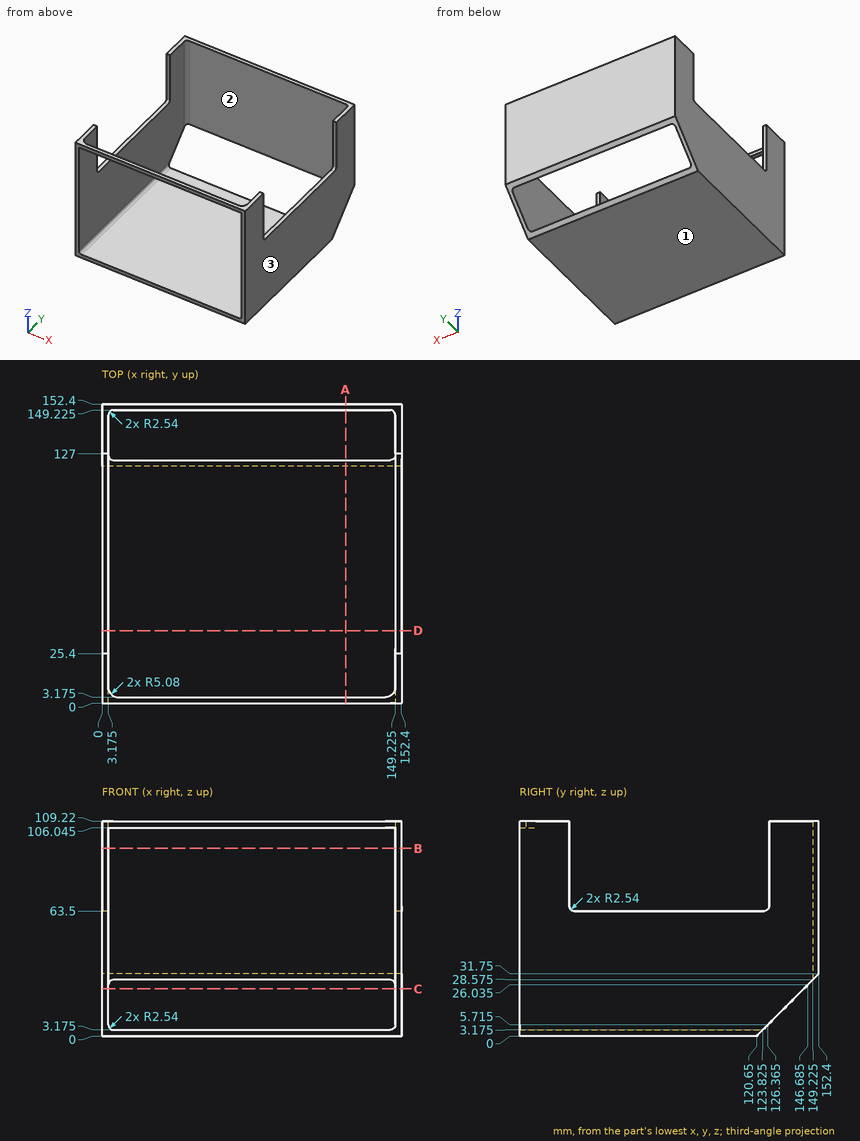
Answer from the drawing. Dimensions are ordinates in mm from the lowest x, y and z of the part. Coordinates: 2 decimals unless noted, no trailing zeros. Loops run counter-clockwise (first coordinate to the right, second up) from the corner with the lowest first, then second, coordinate; pieces in that order, holes last.
Q1. The part is cut by section A-A on x = 124. Write down the section's boundary in (y, z) (3 decimals).
Q2. The part is cut by section C-C on z = 24. Write down the section's boundary in (x, y) (3 decimals).
Q3. Each of these flat-tipped pins is pushed along its axis until it touches: pin 1 Ø2.5 at (x, y) = (1.5, 56) entering from +Z; pin 2 Ø12 at (x, z) = (124.5, 45.5) entering from -Y (3 decimals). Where does it stop, or does it pass through?
Q4. Consider probe 1 along X at (y, z) = (77, 32) (3 decimals); probe 2 along Z at (x, y) = (82.5, 10) (3 decimals); probe 3 along Y at (x, z) = (145, 65) (3 decimals). Determine where each line is inside the solid, lowest interval first.
Q5. The part is cut by section D-D on y = 37. Write down the section's boundary in (x, z) (3 decimals).
Q6. The mould has two halves that part along X. Classify the marked faces 1, 2 and 3: +X half, -X half, draft (parallel to the pull), parting line (faces both ways), or undercut.
Q7. The part is cut by section B-B on z = 95.5. Write down the section's boundary in (x, y) (3 decimals), and give its area (3 significant figures).
Results below:
1. outline: (0, 0) - (120.65, 0) - (123.825, 3.175) - (0, 3.175) - close; (0, 106.045) - (3.175, 106.045) - (3.175, 109.22) - (0, 109.22) - close; (149.225, 28.575) - (152.4, 31.75) - (152.4, 109.22) - (149.225, 109.22) - close
2. outline: (0, 0) - (3.175, 0) - (3.175, 144.65) - (0, 144.65) - close; (149.225, 0) - (152.4, 0) - (152.4, 144.65) - (149.225, 144.65) - close
3. pin 1: stops at z = 63.5
3. pin 2: stops at y = 149.225
4. probe 1: x = 0 to 3.175, 149.225 to 152.4
4. probe 2: z = 0 to 3.175
4. probe 3: y = 149.225 to 152.4
5. outline: (0, 0) - (152.4, 0) - (152.4, 63.5) - (149.225, 63.5) - (149.225, 5.715) arc R2.54 cw to (146.685, 3.175) - (5.715, 3.175) arc R2.54 cw to (3.175, 5.715) - (3.175, 63.5) - (0, 63.5) - close
6. face 1: draft
6. face 2: undercut
6. face 3: +X half
7. outline: (0, 0) - (3.175, 0) - (3.175, 25.4) - (0, 25.4) - close; (0, 127) - (3.175, 127) - (3.175, 146.685) arc R2.54 cw to (5.715, 149.225) - (146.685, 149.225) arc R2.54 cw to (149.225, 146.685) - (149.225, 127) - (152.4, 127) - (152.4, 152.4) - (0, 152.4) - close; (149.225, 0) - (152.4, 0) - (152.4, 25.4) - (149.225, 25.4) - close
7. area: 789 mm2
